Part model, mm, in its own coordinate system. Face numbers are marked on the shaded views. A direction names the side the tool comes from. Round coordinates to 2 decimals unless told otherwise and drop trailing zeros. Write each loop counter-clockwise with the first axis right and the second up, starting at its lowest first coordinate (ties: lowest second). Pieces come first, ordered by that corner, then holes.
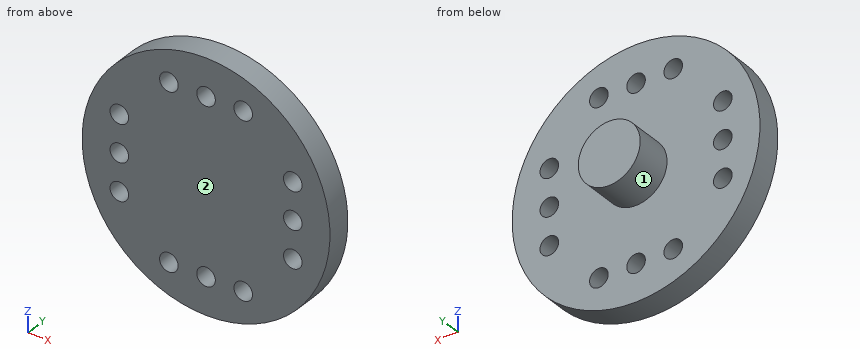
```python
from build123d import *

# Parameters (mm, degrees)
SKETCH_1_R          = 10
EXTRUDE_1_DEPTH     = 2
SKETCH_2_R          = 2.5
EXTRUDE_2_DEPTH     = 3
SKETCH_3_R          = 0.75
CUT_EXTRUDE_1_DEPTH = 15.456832295


with BuildPart() as part:
    # 草图1 → 凸台-拉伸1 (new body)
    with BuildSketch(Plane(origin=(0, 0, 0), x_dir=(1, 0, 0), z_dir=(0, 1, 0))):
        with Locations(Location((0, 0, 0), (0, 0, 270))):
            Circle(SKETCH_1_R)
    extrude(amount=EXTRUDE_1_DEPTH)

    # 草图2 → 凸台-拉伸2 (add)
    with BuildSketch(Plane(origin=(0, 2, 0), x_dir=(1, 0, 0), z_dir=(0, 1, 0))):
        with Locations(Location((0, 0, 0), (0, 0, 270))):
            Circle(SKETCH_2_R)
    extrude(amount=EXTRUDE_2_DEPTH)

    # 草图3 → 切除-拉伸1 (cut, through all)
    with BuildSketch(Plane(origin=(0, 2, 0), x_dir=(1, 0, 0), z_dir=(0, 1, 0))):
        with Locations(Location((0, 7, 0), (0, 0, 270))):
            Circle(SKETCH_3_R)
        with Locations(Location((-3, 7, 0), (0, 0, 270))):
            Circle(SKETCH_3_R)
        with Locations(Location((3, 7, 0), (0, 0, 270))):
            Circle(SKETCH_3_R)
        with Locations(Location((7, 3, 0), (0, 0, 270))):
            Circle(SKETCH_3_R)
        with Locations(Location((7, 0, 0), (0, 0, 270))):
            Circle(SKETCH_3_R)
        with Locations(Location((7, -3, 0), (0, 0, 270))):
            Circle(SKETCH_3_R)
        with Locations(Location((3, -7, 0), (0, 0, 270))):
            Circle(SKETCH_3_R)
        with Locations(Location((0, -7, 0), (0, 0, 270))):
            Circle(SKETCH_3_R)
        with Locations(Location((-3, -7, 0), (0, 0, 270))):
            Circle(SKETCH_3_R)
        with Locations(Location((-7, -3, 0), (0, 0, 270))):
            Circle(SKETCH_3_R)
        with Locations(Location((-7, 0, 0), (0, 0, 270))):
            Circle(SKETCH_3_R)
        with Locations(Location((-7, 3, 0), (0, 0, 270))):
            Circle(SKETCH_3_R)
    extrude(amount=-CUT_EXTRUDE_1_DEPTH, mode=Mode.SUBTRACT)


solid = part.part
```
Q1. Which spindle directions (+Z, -Z, +X, -X, +Y, -Y) get a long thin tool onto all of the face, cutting with end or side? Do the marked faces 1 and 2. Say none if no direction does.
Values follow:
face 1: +Y
face 2: +Z, -Z, +X, -X, -Y
Q2. Cut at C-C on x = -7. Write the cut outline in (y, z).
Values follow:
outline: (0, -7.14) - (2, -7.14) - (2, -3.75) - (0, -3.75) - close; (0, -2.25) - (2, -2.25) - (2, -0.75) - (0, -0.75) - close; (0, 0.75) - (2, 0.75) - (2, 2.25) - (0, 2.25) - close; (0, 3.75) - (2, 3.75) - (2, 7.14) - (0, 7.14) - close
Q3. Cut at D-D on z = -7. Write the cut outline in (x, y).
Values follow:
outline: (-7.14, 0) - (-3.75, 0) - (-3.75, 2) - (-7.14, 2) - close; (-2.25, 0) - (-0.75, 0) - (-0.75, 2) - (-2.25, 2) - close; (0.75, 0) - (2.25, 0) - (2.25, 2) - (0.75, 2) - close; (3.75, 0) - (7.14, 0) - (7.14, 2) - (3.75, 2) - close
Q4. Drop flat-ended pins along their axis: pin 1 (1.5 mm diameter, centred on x = 4.5, z = -6, fed in from +Y); pin 2 (1.2 mm diameter, centred on x = -3, z = -7, fed in from -Y); pin 3 (2 mm diameter, centred on y = 2.5, z = 5.5, fed in from +X). Give the stop position or say it passes through.
Values follow:
pin 1: stops at y = 2
pin 2: passes through
pin 3: stops at x = 8.86
Q5. Cut at B-B on z = 0. Write the cut outline in (x, y).
Values follow:
outline: (-10, 0) - (-7.75, 0) - (-7.75, 2) - (-10, 2) - close; (-6.25, 0) - (6.25, 0) - (6.25, 2) - (2.5, 2) - (2.5, 5) - (-2.5, 5) - (-2.5, 2) - (-6.25, 2) - close; (7.75, 0) - (10, 0) - (10, 2) - (7.75, 2) - close
Q6. Cut at A-A on y = 1.3. State how many separate pieces and enclosed holes the cut face has, plus the area to 3 significant figures.
Values follow:
separate pieces: 1
enclosed holes: 12
area: 293 mm2
Q7. Wall check: L1, parallel to X at y = 0.5, z = 0; L2, parallel to X at y = 1.5, z = -7; L3, parallel to X at y = 0.75, z = 3. Give the ranges that are in metal, low to high.
Values follow:
L1: x = -10 to -7.75, -6.25 to 6.25, 7.75 to 10
L2: x = -7.14 to -3.75, -2.25 to -0.75, 0.75 to 2.25, 3.75 to 7.14
L3: x = -9.54 to -7.75, -6.25 to 6.25, 7.75 to 9.54
